```python
from build123d import *

# Parameters (mm, degrees)
BOX001_W     = 280
BOX001_H     = 280
BOX001_DEPTH = 5
SKETCH_W     = 300
SKETCH_H     = 300
SKETCH_W_2   = 280
SKETCH_H_2   = 280
PAD_DEPTH    = 15


with BuildPart() as cube001:
    # Box001 → Box001 (new body)
    with BuildSketch(Plane(origin=(-140, -140, 0), x_dir=(1, 0, 0), z_dir=(0, 0, 1))):
        with Locations((140, 140)):
            Rectangle(BOX001_W, BOX001_H)
    extrude(amount=BOX001_DEPTH)


with BuildPart() as board_frame:
    # Sketch → Pad (new body)
    with BuildSketch(Plane.XY):
        Rectangle(SKETCH_W, SKETCH_H)
        Rectangle(SKETCH_W_2, SKETCH_H_2, mode=Mode.SUBTRACT)
    extrude(amount=PAD_DEPTH)

    # Fusion: union Cube001
    add(cube001.part)


solid = board_frame.part
```
CAD build for the part. Positions are in the model's coordinates, mm. A direction names the side the tool comes from. Give positions to 0.01 mm unless a question says otherwise; leave off trailing zeros. Loops run counter-clockwise (first coordinate to the right, second up) from the corner with the lowest first, then second, coordinate; pieces in that order, holes last. Notation, with made-up numbers: M 28,29.25 L 48,29.25 A33 ccw 48,59.25 Z; hole C 67.25,13.25 d9. An arc over 180 degrees is marked long. Use one line per item in the form item = value.
Item 1: Slice it at A-A (z = 9.5). List the corners of the cut face in (x, y).
Determined:
outline = M -150,-150 L 150,-150 L 150,150 L -150,150 Z; hole M -140,-140 L 140,-140 L 140,140 L -140,140 Z
Item 2: Slice it at B-B (y = 103). List the corners of the cut face in (x, z), plus the area to 3 significant figures.
Determined:
outline = M -150,0 L 150,0 L 150,15 L 140,15 L 140,5 L -140,5 L -140,15 L -150,15 Z
area = 1,700 mm2
Item 3: Flat gauge pin, fed straight in: pin 1 (10 mm diameter, centred on x = 60, y = 46, fed in from +Z). Where does the tip first touch, or does it go through?
Determined:
pin_1 = 5
Item 4: Drill centre lines: probe 1 along X at (y, z) = (-64, 9); probe 2 along Z at (x, y) = (103.5, -8.5). Where is each one in solid material? Low to high. Write a range as from..to.
Determined:
probe_1 = -150..-140, 140..150
probe_2 = 0..5
Item 5: Which spindle directions (+Z, -Z, +X, -X, +Y, -Y) get a long thin tool onto all of the face, cutting with end or side? Do faces 1 (the face through (-140, -2, 10)), 2 (the face through (-12, -144, 15)). Say none if no direction does.
Determined:
face_1 = +Z
face_2 = +Z, +X, -X, +Y, -Y
Item 6: Two-plate mould, pull along Y, no slides. Class faces 3 (the face through (150, -2, 7)), 4 (the face through (-2, 150, 7)), 5 (the face through (140, -2, 10)): pulls with the +Y half, pulls with the -Y half, needs draft (parallel to the pull), parting line crosses it, or undercut.
Determined:
face_3 = needs draft
face_4 = pulls with the +Y half
face_5 = undercut
